from build123d import *

# Parameters (mm, degrees)
SKETCH1_W           = 70
SKETCH1_H           = 10
BOSS_EXTRUDE1_DEPTH = 2
CUT_EXTRUDE1_START  = -5
CUT_EXTRUDE1_DEPTH  = 2.8
CUT_EXTRUDE2_START  = -47
CUT_EXTRUDE2_DEPTH  = 2.8
SKETCH3_W           = 15
SKETCH3_H           = 10
CUT_EXTRUDE3_DEPTH  = 1
SKETCH4_W           = 8
SKETCH4_H           = 6
CUT_EXTRUDE4_DEPTH  = 36.369478368


with BuildPart() as part:
    # Sketch1 → Boss-Extrude1 (new body)
    with BuildSketch(Plane(origin=(0, 0, 0), x_dir=(1, 0, 0), z_dir=(0, 1, 0))):
        Rectangle(SKETCH1_W, SKETCH1_H)
    extrude(amount=BOSS_EXTRUDE1_DEPTH)

    # Sketch2 → Cut-Extrude1 (cut)
    with BuildSketch(Plane(origin=(35, 0, 0), x_dir=(0, 0, -1), z_dir=(1, 0, 0)).offset(CUT_EXTRUDE1_START)):
        Polygon((-5, 2), (-5, 1), (-4, 2), align=None)
        Polygon((5, 2), (5, 1), (4, 2), align=None)
    extrude(amount=-CUT_EXTRUDE1_DEPTH, mode=Mode.SUBTRACT)

    # Sketch2<2> → Cut-Extrude2 (cut)
    with BuildSketch(Plane(origin=(35, 0, 0), x_dir=(0, 0, -1), z_dir=(1, 0, 0)).offset(CUT_EXTRUDE2_START)):
        Polygon((-5, 2), (-5, 1), (-4, 2), align=None)
        Polygon((5, 2), (5, 1), (4, 2), align=None)
    extrude(amount=-CUT_EXTRUDE2_DEPTH, mode=Mode.SUBTRACT)

    # Sketch3 → Cut-Extrude3 (cut)
    with BuildSketch(Plane.XZ):
        with Locations((-27.5, 0)):
            Rectangle(SKETCH3_W, SKETCH3_H)
    extrude(amount=-CUT_EXTRUDE3_DEPTH, mode=Mode.SUBTRACT)

    # Sketch4 → Cut-Extrude4 (cut, through all)
    with BuildSketch(Plane.XZ.offset(-1)):
        with Locations((-27.5, 0)):
            Rectangle(SKETCH4_W, SKETCH4_H)
    extrude(amount=-CUT_EXTRUDE4_DEPTH, mode=Mode.SUBTRACT)


solid = part.part
Could you check a few things on this model? Use its own coordinates, in mm. A direction names the side the tool comes from. Round coordinates to 2 decimals unless told otherwise and drop trailing zeros. Write each loop counter-clockwise with the first axis right and the second up, starting at its lowest first coordinate (ties: lowest second). Pieces come first, ordered by that corner, then holes. Notation, with made-up numbers: (69.25, 72.5) -> (104.25, 72.5) arc R24 cw to (104.25, 98.5) -> close; hole circle Ø4 at (63, -19). An arc over 180 degrees is marked (long way). Use a Markdown table: item, result.
1. Please list where these lines run through material, in increasing order: probe 1 along X at (y, z) = (1.45, -1.5); probe 2 along Z at (x, y) = (-28, 1.75); probe 3 along X at (y, z) = (0.65, -3).
Answer key:
| item | result |
|---|---|
| probe 1 | x = -35 to -31.5, -23.5 to 35 |
| probe 2 | z = -5 to -3, 3 to 5 |
| probe 3 | x = -20 to 35 |
2. Which directions (+Z, -Z, +X, -X, +Y, -Y) give clear straight access to the entire face, cutting with the end or side of a thin tool? Please do faces 1 (the face through (-27.6, 1, 3.4)), 2 (the face through (7, 0, 0)).
Answer key:
| item | result |
|---|---|
| face 1 | +Z, -Z, -X, -Y |
| face 2 | +Z, -Z, +X, -X, -Y |
3. For pin 1 Ø0.5 at (y, z) = (0.5, -2) entering from -X; pin 2 Ø4 at (x, z) = (-12, 3) entering from -Y, each with a flat end and sliding along its axis, tell me the tip position at first contact or that it passes through.
Answer key:
| item | result |
|---|---|
| pin 1 | stops at x = -20 |
| pin 2 | stops at y = 0 |
4. If we section it at C-C (z = 0.25): List the corners of the cut face in (x, y) for me.
Answer key:
| item | result |
|---|---|
| outline | (-35, 1) -> (-31.5, 1) -> (-31.5, 2) -> (-35, 2) -> close; (-23.5, 1) -> (-20, 1) -> (-20, 0) -> (35, 0) -> (35, 2) -> (-23.5, 2) -> close |
5. If we section it at B-B (x = -29): List the corners of the cut face in (y, z) for me, then the cut area to 3 significant figures.
Answer key:
| item | result |
|---|---|
| outline | (1, -5) -> (2, -5) -> (2, -3) -> (1, -3) -> close; (1, 3) -> (2, 3) -> (2, 5) -> (1, 5) -> close |
| area | 4.00 mm^2 |
6. If we section it at A-A (y = 1.7): List the corners of the cut face in (x, z) for me.
Answer key:
| item | result |
|---|---|
| outline | (-35, -5) -> (-14.8, -5) -> (-14.8, -4.3) -> (-12, -4.3) -> (-12, -5) -> (27.2, -5) -> (27.2, -4.3) -> (30, -4.3) -> (30, -5) -> (35, -5) -> (35, 5) -> (30, 5) -> (30, 4.3) -> (27.2, 4.3) -> (27.2, 5) -> (-12, 5) -> (-12, 4.3) -> (-14.8, 4.3) -> (-14.8, 5) -> (-35, 5) -> close; hole (-31.5, -3) -> (-23.5, -3) -> (-23.5, 3) -> (-31.5, 3) -> close |
